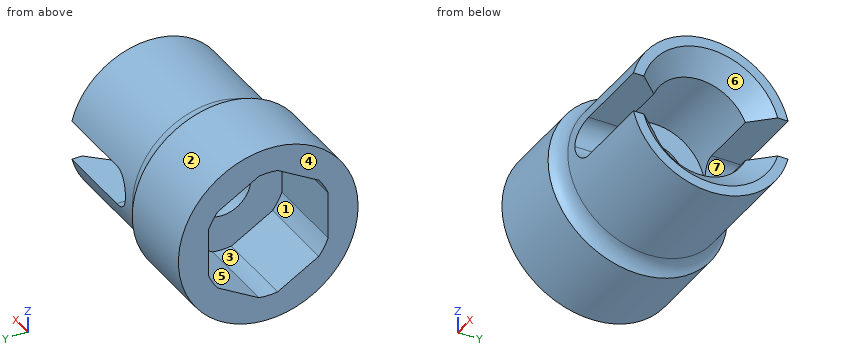
from build123d import *

# Parameters (mm, degrees)
SKETCH1_W               = 25.4
SKETCH1_H               = 3.175
SKETCH1_W_2             = 1.5875
SKETCH1_H_2             = 1.5875
SKETCH1_W_3             = 7.9375
SKETCH1_H_3             = 2.38125
CUT_EXTRUDE1_DEPTH      = 27.940768363
CUT_EXTRUDE1_DEPTH_BACK = 27.940768363
SKETCH2_W               = 0.79375
SKETCH2_H               = 3.175
SKETCH2_R               = 1.5875
FILLET1_R               = 1.5875
CHAMFER1_SIZE           = 1.5875
CUT_EXTRUDE2_DEPTH      = 27.94076841
SKETCH3_3_R             = 2.286
CUT_EXTRUDE3_DEPTH      = 14.67923997
SKETCH3_4_R             = 7.14375
BOSS_EXTRUDE1_DEPTH     = 6.5405
FILLET2_R               = 1.5875


# Some blends are built 0.0001 mm under size
with BuildPart() as part:
    # Sketch1 → Revolve1 (revolve)
    with BuildSketch(Plane.XY):
        with Locations((-12.7, 1.5875)):
            Rectangle(SKETCH1_W, SKETCH1_H)
        with Locations((-0.79375, 3.96875)):
            Rectangle(SKETCH1_W_2, SKETCH1_H_2)
        Polygon((0, 3.175), (0, 0), (2.38125, 0), (2.38125, 3.96875), (2.38125, 6.35), (0, 6.35), (0, 4.7625), align=None)
        with Locations((6.35, 5.159375)):
            Rectangle(SKETCH1_W_3, SKETCH1_H_3)
    revolve(axis=Axis((0, 0, 0), (-1, 0, 0)))

    # Sketch2 → Cut-Extrude1 (cut, two sides: drawn at the far end of the back side and taken through both)
    with BuildSketch(Plane(origin=(0, 0, 0), x_dir=(1, 0, 0), z_dir=(0, 1, 0)).offset(-CUT_EXTRUDE1_DEPTH_BACK)):
        with Locations((2.778125, 0)):
            Rectangle(SKETCH2_W, SKETCH2_H)
        with BuildLine():
            Line((3.175, -1.5875), (6.35, -1.5875))
            ThreePointArc((6.35, -1.5875), (4.7625, 0), (6.35, 1.5875))
            Line((6.35, 1.5875), (3.175, 1.5875))
            Line((3.175, 1.5875), (3.175, -1.5875))
        make_face()
        with Locations((6.35, 0)):
            Circle(SKETCH2_R)
        with BuildLine():
            Line((6.35, -1.5875), (10.31875, -1.5875))
            Line((10.31875, -1.5875), (10.31875, 1.5875))
            Line((10.31875, 1.5875), (6.35, 1.5875))
            ThreePointArc((6.35, 1.5875), (7.472532015, 1.122532015), (7.9375, 0))
            ThreePointArc((7.9375, 0), (7.472532015, -1.122532015), (6.35, -1.5875))
        make_face()
    extrude(amount=CUT_EXTRUDE1_DEPTH + CUT_EXTRUDE1_DEPTH_BACK, mode=Mode.SUBTRACT)

    # Fillet1
    fillet1_edges = [part.edges().sort_by_distance(p)[0] for p in [
        (2.38125, -4.89289026, -1.5875),
        (2.38125, 4.89289026, -1.5875),
        (2.38125, -4.89289026, 1.5875),
        (2.38125, 4.89289026, 1.5875),
    ]]
    fillet(fillet1_edges, radius=FILLET1_R - 0.0001)  # a hair under: the kernel refuses the full size

    # Chamfer1
    chamfer1_edges = [part.edges().sort_by_distance(p)[0] for p in [
        (10.31875, 0, 3.96875),
        (10.31875, 0, -3.96875),
    ]]
    chamfer(chamfer1_edges, length=CHAMFER1_SIZE)

    # Sketch3 → Cut-Extrude2 (cut, through all)
    with BuildSketch(Plane.ZY):
        with BuildLine():
            Line((-5.034429311, 5.567612646), (-7.338908645, 1.576137354))
            ThreePointArc((-7.338908645, 1.576137354), (-7.50625, 0), (-7.338908645, -1.576137354))
            Line((-7.338908645, -1.576137354), (-5.034429311, -5.567612646))
            ThreePointArc((-5.034429311, -5.567612646), (-3.753125, -6.500603187), (-2.304479334, -7.14375))
            Line((-2.304479334, -7.14375), (2.304479334, -7.14375))
            ThreePointArc((2.304479334, -7.14375), (3.753125, -6.500603187), (5.034429311, -5.567612646))
            Line((5.034429311, -5.567612646), (7.338908645, -1.576137354))
            ThreePointArc((7.338908645, -1.576137354), (7.50625, 0), (7.338908645, 1.576137354))
            Line((7.338908645, 1.576137354), (5.034429311, 5.567612646))
            ThreePointArc((5.034429311, 5.567612646), (3.753125, 6.500603187), (2.304479334, 7.14375))
            Line((2.304479334, 7.14375), (-2.304479334, 7.14375))
            ThreePointArc((-2.304479334, 7.14375), (-3.753125, 6.500603187), (-5.034429311, 5.567612646))
        make_face()
    extrude(amount=CUT_EXTRUDE2_DEPTH, mode=Mode.SUBTRACT)

    # Sketch3<3> → Cut-Extrude3 (cut, through all)
    with BuildSketch(Plane.ZY):
        with Locations(Location((0, 0, 0), (0, 0, 270))):
            Circle(SKETCH3_3_R)
    extrude(amount=-CUT_EXTRUDE3_DEPTH, mode=Mode.SUBTRACT)

    # Sketch3<4> → Boss-Extrude1 (add)
    with BuildSketch(Plane.ZY):
        with Locations(Location((0, 0, 0), (0, 0, 270))):
            Circle(SKETCH3_4_R)
        with BuildLine():
            Line((3.177844334, -4.020812156), (5.071047637, -0.741687844))
            ThreePointArc((5.071047637, -0.741687844), (5.125, 0), (5.071047637, 0.741687844))
            Line((5.071047637, 0.741687844), (3.177844334, 4.020812156))
            ThreePointArc((3.177844334, 4.020812156), (2.5625, 4.438380194), (1.893203304, 4.7625))
            Line((1.893203304, 4.7625), (-1.893203304, 4.7625))
            ThreePointArc((-1.893203304, 4.7625), (-2.5625, 4.438380194), (-3.177844334, 4.020812156))
            Line((-3.177844334, 4.020812156), (-5.071047637, 0.741687844))
            ThreePointArc((-5.071047637, 0.741687844), (-5.125, 0), (-5.071047637, -0.741687844))
            Line((-5.071047637, -0.741687844), (-3.177844334, -4.020812156))
            ThreePointArc((-3.177844334, -4.020812156), (-2.5625, -4.438380194), (-1.893203304, -4.7625))
            Line((-1.893203304, -4.7625), (1.893203304, -4.7625))
            ThreePointArc((1.893203304, -4.7625), (2.5625, -4.438380194), (3.177844334, -4.020812156))
        make_face(mode=Mode.SUBTRACT)
    extrude(amount=BOSS_EXTRUDE1_DEPTH)

    # Fillet2
    # the kernel refuses this fillet: 1.5875 mm, written as the material it adds along each edge
    with BuildSketch(Plane(origin=(0, 0, 0), x_dir=(0, 1, 0), z_dir=(0, 0, 1))) as fillet2_piece_1:
        with BuildLine():
            CenterArc((7.9375, -1.374815329), FILLET2_R, 120, 60)
            Line((7.14375, 0), (7.127875, 0.027496307))
            ThreePointArc((7.127875, 0.027496307), (6.746875, 0.03175), (6.35, 0.03175))
            Line((6.35, 0.03175), (6.31825, 0))
            Line((6.31825, 0), (6.31825, -1.374815329))
            Line((6.31825, -1.374815329), (6.35, -1.374815329))
        make_face()
    revolve(axis=Axis((0, 0, 0), (-1, 0, 0)))


solid = part.part
CAD build for the part. Positions are in the model's coordinates, mm. Face numbers are marked on the shaded views. A direction names the side the tool comes from. Round coordinates to 2 decimals unless told otherwise and drop trailing zeros. Write each loop counter-clockwise with the first axis right and the second up, starting at its lowest first coordinate (ties: lowest second). Pieces come first, ordered by that corner, then holes. Notation, with made-up numbers: M 27.25,57.25 L 61.25,57.25 A15 cw 61.25,71.25 Z; hole C -36.75,25.5 d4. An arc over 180 degrees is marked long. Put each result on its own line as item: value. Start each with the question number.
1) Saw through at A-A, the plane x = 7.75. Write the cut outline in (y, z), and give its area (3 significant figures).
2) Drill centre lines: probe 1 along Z at (x, y) = (1.7, 0); probe 2 along Z at (x, y) = (1, 0); probe 3 along Y at (x, z) = (5, -5.5). Where is each one in solid material? Low to high. Write a range as [from, to].
3) Pull direction Z, two halves, no side cores. Call the marked faces 1, 2, 3 and 4: pulls with the +Z half, pulls with the -Z half, needs draft (parallel to the pull), parting line crosses it, or undercut.
4) Pin check, flat tips, straight feed: pin 1 Ø2 at (x, y) = (7.5, -4.5) entering from -Z; pin 2 Ø3 at (x, y) = (7.5, -5.5) entering from +Z; pin 3 Ø3 at (x, z) = (-3, 4.5) entering from -Y. Stop position of each tip, or through.
5) 3-axis set-ups, long thin cutter, end or side, ignore diameter. For the marked faces 5, 6 and 7: which of +Z, -Z, +X, -X, +Y, -Y reach the whole face in a straight line?
Resolved:
1. outline: M -6.15,-1.59 A6.35 ccw 6.15,-1.59 L 3.64,-1.59 A3.97 cw -3.64,-1.59 Z; M -6.15,1.59 L -3.64,1.59 A3.97 cw 3.64,1.59 L 6.15,1.59 A6.35 ccw Z
1. area: 61.8 mm²
2. probe 1: [-6.35, -2.29], [2.29, 6.35]
2. probe 2: [-6.39, -2.29], [2.29, 6.39]
2. probe 3: [-3.17, 3.17]
3. face 1: undercut
3. face 2: parting line crosses it
3. face 3: undercut
3. face 4: needs draft
4. pin 1: z = -5.3
4. pin 2: z = 4.93
4. pin 3: y = -6.48
5. face 5: -X
5. face 6: +X
5. face 7: +X, +Y, -Y
